Geometry: final body of the model. Coordinates: model frame, mm. A direction names the side the tool comes from. Give positions to 0.01 mm unless a question says otherwise; leave off trailing zeros. Write each loop counter-clockwise with the first axis right and the second up, starting at its lowest first coordinate (ties: lowest second). Pieces come first, ordered by that corner, then holes. Notation, with made-up numbers: M 18.5,20 L 41.5,20 A31 cw 41.5,58 Z; hole C 40,35 d8. An arc over 180 degrees is marked long. One line per question, with ' | ' between items.
from build123d import *

# Parameters (mm, degrees)
SKETCH1_R           = 1.5
BOSS_EXTRUDE1_DEPTH = 2.7


with BuildPart() as part:
    # Sketch1 → Boss-Extrude1 (new body)
    with BuildSketch(Plane(origin=(0, 0, 0), x_dir=(1, 0, 0), z_dir=(0, 1, 0))):
        Polygon((4, 2.833333333), (4, 12.366666667), (6.7, 12.366666667), (6.7, 21.9), (4, 21.9), (4, 19.2), (-36.5, 19.2), (-36.5, 21.9), (-77, 21.9), (-77, 19.2), (-117.5, 19.2), (-117.5, 12.366666667), (-117.5, 2.833333333), (-117.5, -4), (-77, -4), (-77, -6.7), (-36.5, -6.7), (-36.5, -4), (4, -4), (4, -6.7), (6.7, -6.7), (6.7, 2.833333333), align=None)
        with Locations((-3.5, 6.3)):
            Circle(SKETCH1_R, mode=Mode.SUBTRACT)
        with Locations((-60.7, 6.3)):
            Circle(SKETCH1_R, mode=Mode.SUBTRACT)
        with Locations((-92.8, 5.7)):
            Circle(SKETCH1_R, mode=Mode.SUBTRACT)
    extrude(amount=BOSS_EXTRUDE1_DEPTH)


solid = part.part
(1) First-contact query: P1, Ø0.8, axis at x = -17.5, y = 1, coming from the +Z side. Flat tip, straight axial feed; report the tip coordinate or a pass-through.
Working result:
P1: stops at z = 4
(2) Cut plane C-C, the plane x = -60.7. Return loops of the section in (y, z), then the cut area to 3 significant figures.
Working result:
outline: M 0,-21.9 L 2.7,-21.9 L 2.7,-7.8 L 0,-7.8 Z; M 0,-4.8 L 2.7,-4.8 L 2.7,6.7 L 0,6.7 Z | area: 69.1 mm^2
(3) Material intervals for L1, parallel to Z at x = -3.5, y = 1.3; L2, parallel to X at y = 1.1, z = -6.3; L3, parallel to Z at x = -21, y = 2.5, sorted ascending. Write a range as [from, to].
Working result:
L1: z = [-19.2, -7.8], [-4.8, 4] | L2: x = [-117.5, -94.17], [-91.43, -62.2], [-59.2, -5], [-2, 4] | L3: z = [-19.2, 4]
(4) Draft query along X for faces 6 (the face through (4, 1, -21)), 7 (the face through (-117.5, 1, -8)), 8 (the face through (4, 1, -8)). Return one class per face: released by +X, released by -X, zero draft, split by the parting line, or undercut.
Working result:
face 6: undercut | face 7: released by -X | face 8: released by +X
(5) Cut plane B-B, the plane y = 0.65. Return loops of the section in (x, z), then the cut area to 3 significant figures.
Working result:
outline: M -117.5,-19.2 L -77,-19.2 L -77,-21.9 L -36.5,-21.9 L -36.5,-19.2 L 4,-19.2 L 4,-21.9 L 6.7,-21.9 L 6.7,-12.37 L 4,-12.37 L 4,-2.83 L 6.7,-2.83 L 6.7,6.7 L 4,6.7 L 4,4 L -36.5,4 L -36.5,6.7 L -77,6.7 L -77,4 L -117.5,4 Z; hole C -92.8,-5.7 d3; hole C -60.7,-6.3 d3; hole C -3.5,-6.3 d3 | area: 3,070 mm^2
(6) Cut plane A-A, the plane x = -3.5. Return loops of the section in (y, z), then the cut area to 3 significant figures.
Working result:
outline: M 0,-19.2 L 2.7,-19.2 L 2.7,-7.8 L 0,-7.8 Z; M 0,-4.8 L 2.7,-4.8 L 2.7,4 L 0,4 Z | area: 54.5 mm^2
(7) Set-up query: faces 1 (the face through (-56, 1, -21.9)), 2 (the face through (-77, 1, 5)), 3 (the face through (-36.5, 1, 5)), 4 (the face through (-36.5, 1, -21)), 5 (the face through (5, 1, -2.833)). Return all of +Z, -Z, +X, -X, +Y, -Y with unobstructed straight access to the full face (end or side cutting, diameter ignored); none if empty.
Working result:
face 1: -Z, +X, -X, +Y, -Y | face 2: +Z, -X, +Y, -Y | face 3: +Z, +Y, -Y | face 4: -Z, +Y, -Y | face 5: +X, +Y, -Y
